Can you work these out from the model? Positions are in its coordinate system, mm. Face numbers are marked on the shaded views. A direction names the side the tool comes from. Coordinates: 2 decimals unless noted, no trailing zeros. Order: outer loops, then holes, each group sorted by start corner. A loop starts at its lowest first (then second) coordinate and runs counter-clockwise, first axis right, second up. Notation, with made-up numbers: (88.25, -23.75) -> (116.25, -23.75) arc R15 ccw to (116.25, 4.25) -> close; hole circle Ø1 at (31.5, 30.25). An arc over 180 degrees is marked (long way). Return JSON: item names as keys, results as strings. Group by question number.
1) If we section it at B-B, the plane z = 3: Please give me the cut outline in (x, y).
2) If we section it at C-C, the plane x = 24: Please give me the cut outline in (y, z).
3) Thinking about a two-plate mould opening in X: for the marked faces 3, 4 and 5, which applies, +X half, -X half, draft (parallel to the pull), parting line (faces both ways), or undercut?
4) If I drill on probe 1 along Z at (x, y) = (0, 2.25); probe 2 along X at (y, z) = (1, 0.5); probe 3 along Z at (x, y) = (26.5, 1), over which ranges is the centre line in solid material (lowest first)? Write a range as from..to.
5) For pin 1 (1 mm diameter, centred on x = 28, y = 8, fed in from +Z); pin 2 (1.2 mm diameter, centred on x = 0, z = 0, fed in from +Y); pin 3 (5 mm diameter, centred on y = 6, z = 3.5, fed in from +X), each with a flat end and sliding along its axis, tell me the tip position at first contact or that it passes through.
6) If we section it at D-D, the plane z = 9.5: Please give me the cut outline in (x, y), then the cut area to 3 significant figures.
7) For the marked faces 1 and 2, which set-ups out of +Z, -Z, +X, -X, +Y, -Y let a thin tool reach every point of the face, with its end or its side?
8) If we section it at A-A, the plane y = 9.25: Please give me the cut outline in (x, z).
from build123d import *

# Parameters (mm, degrees)
BOSS_EXTRUDE2_DEPTH = 10


with BuildPart() as part:
    # Sketch1 → Boss-Extrude2 (new body)
    with BuildSketch(Plane(origin=(0, 0, 0), x_dir=(1, 0, 0), z_dir=(0, 1, 0))):
        with BuildLine():
            ThreePointArc((12.410397071, 0), (8.775475926, 8.775475926), (0, 12.410397071))
            Line((0, 12.410397071), (0, 1))
            ThreePointArc((0, 1), (0.707106781, 0.707106781), (1, 0))
            Line((1, 0), (12.410397071, 0))
        make_face()
        with BuildLine():
            Line((0, 1), (0, 12.410397071))
            ThreePointArc((0, 12.410397071), (-8.775475926, -8.775475926), (12.410397071, 0))
            Line((12.410397071, 0), (1, 0))
            ThreePointArc((1, 0), (-0.707106781, -0.707106781), (0, 1))
        make_face()
        with BuildLine():
            Line((30.017427339, 12.410397071), (0, 12.410397071))
            ThreePointArc((0, 12.410397071), (8.775475926, 8.775475926), (12.410397071, 0))
            Line((12.410397071, 0), (30.017427339, 0))
            Line((30.017427339, 0), (30.017427339, 12.410397071))
        make_face()
        Polygon((30.017427339, 0), (30.017427339, 12.410397071), (39.086451676, 12.410397071), (56.824436842, -5.327588094), (35.345015433, -5.327588094), align=None)
    extrude(amount=BOSS_EXTRUDE2_DEPTH)


solid = part.part
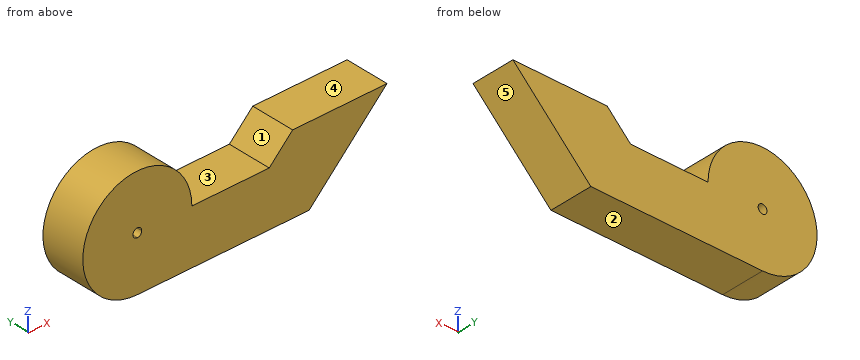
Result sheet:
{
 "1": {"outline": "(-12.04, 0) -> (12.04, 0) -> (12.04, 10) -> (-12.04, 10) -> close; (33.02, 0) -> (54.5, 0) -> (54.5, 10) -> (33.02, 10) -> close"},
 "2": {"outline": "(0, -12.41) -> (10, -12.41) -> (10, 0) -> (0, 0) -> close"},
 "3": {"face 3": "undercut", "face 4": "draft", "face 5": "+X half"},
 "4": {"probe 1": "z = -12.41..-1, 1..12.41", "probe 2": "x = -12.4..-0.87, 0.87..12.4, 30.52..52", "probe 3": "z = -12.41..0"},
 "5": {"pin 1": "stops at z = 0", "pin 2": "passes through", "pin 3": "stops at x = 56.82"},
 "6": {"outline": "(-7.99, 0) -> (7.99, 0) -> (7.99, 10) -> (-7.99, 10) -> close", "area": "160 mm2"},
 "7": {"face 1": "+Z, +Y, -Y", "face 2": "-Z, +X, -X, +Y, -Y"},
 "8": {"outline": "(0, -12.41) -> (39.09, -12.41) -> (56.82, 5.33) -> (35.35, 5.33) -> (30.02, 0) -> (12.41, 0) arc R12.41 ccw (long way) to start; hole circle Ø2 at (0, 0)"}
}
